For this review, take the finished solid that the model builds, in its own axes (mm). A direction names the side the tool comes from. Give positions to 0.01 mm unless a question says otherwise; leave off trailing zeros. Write each loop counter-clockwise with the first axis right and the second up, starting at its lowest first coordinate (ties: lowest second). Pieces come first, ordered by that corner, then holes. Notation, with made-up numbers: M 76,81.25 L 103,81.25 A28 cw 103,114.25 Z; hole C 24.5,43.25 d3. An arc over 180 degrees is marked long. Use one line per item in the form item = value. Start each with the question number.
Q1. Consider section C-C on x = 49. Write out the cut boundary in (y, z).
Q2. Clearance check with flat-ended pins moving along their axes: pin 1 Ø8 at (x, z) = (40.5, 31) entering from +Y; pin 2 Ø10 at (x, y) = (13.5, 5.5) entering from +Z. State where each tip first meets the part, or that it passes through.
Q3. Consider section A-A on z = 4. Write out the cut boundary in (x, y), and give its area (3 significant figures).
Q4. Consider section D-D on z = 21.5. Write out the cut boundary in (x, y) (1 decimal).
Q5. For probe 1 along Y at (x, z) = (35, 38); probe 2 along Y at (x, z) = (63, 31); probe 3 along X at (y, z) = (28, 43), list the stretches that pass through material, from the lowest coordinate up. Write a range as [from, to].
Q6. Consider section B-B on y = 6. Write out the cut boundary in (x, z).
Q7. Tool access review of faces 1 (the flat face through (55, 40, 34)), 2 (the flat face through (32.36, 24.72, 37.78)), 3 (the flat face through (50, 20, 50)): name each direction out of +Z, -Z, +X, -X, +Y, -Y from which nothing blocks a thin tool from reaching the whole face with its end or side.
```python
from build123d import *

# Parameters (mm, degrees)
SKETCH1_W            = 70
SKETCH1_H            = 50
BOSS_EXTRUDE1_DEPTH  = 50
CUT_EXTRUDE1_DEPTH   = 50
CUT_EXTRUDE2_DEPTH   = 81
CUT_EXTRUDE4_DEPTH   = 30
BOSS_EXTRUDE4_DEPTH  = 73
SKETCH7_W            = 70
SKETCH7_H            = 50
CUT_EXTRUDE5_DEPTH   = 73
SKETCH8_W            = 70
SKETCH8_H            = 50
CUT_EXTRUDE6_DEPTH   = 73
CUT_EXTRUDE7_DEPTH   = 73
CUT_EXTRUDE8_DEPTH   = 73
CUT_EXTRUDE9_DEPTH   = 73
CUT_EXTRUDE10_DEPTH  = 73
CUT_EXTRUDE11_DEPTH  = 73
CUT_EXTRUDE12_DEPTH  = 73
CUT_EXTRUDE13_DEPTH  = 73
CUT_EXTRUDE14_DEPTH  = 73
CUT_EXTRUDE15_DEPTH  = 73
CUT_EXTRUDE16_DEPTH  = 73
CUT_EXTRUDE17_DEPTH  = 73
BOSS_EXTRUDE6_DEPTH  = 40
BOSS_EXTRUDE9_DEPTH  = 20
CUT_EXTRUDE18_DEPTH  = 20
CUT_EXTRUDE19_DEPTH  = 20
CUT_EXTRUDE20_DEPTH  = 20
CUT_EXTRUDE21_DEPTH  = 20
CUT_EXTRUDE22_DEPTH  = 20
SKETCH28_W           = 25
SKETCH28_H           = 30
BOSS_EXTRUDE10_DEPTH = 20
CUT_EXTRUDE23_DEPTH  = 20
BOSS_EXTRUDE12_DEPTH = 10
CUT_EXTRUDE24_DEPTH  = 10
CUT_EXTRUDE25_DEPTH  = 10
CUT_EXTRUDE28_DEPTH  = 10
BOSS_EXTRUDE14_DEPTH = 35


with BuildPart() as part:
    # Sketch1 → Boss-Extrude1 (new body)
    with BuildSketch(Plane.XY):
        with Locations((35, 25)):
            Rectangle(SKETCH1_W, SKETCH1_H)
    extrude(amount=BOSS_EXTRUDE1_DEPTH)

    # Sketch2 → Cut-Extrude1 (cut)
    with BuildSketch(Plane.XY.offset(50)):
        Polygon((20, 50), (0, 30), (0, 50), align=None)
    extrude(amount=-CUT_EXTRUDE1_DEPTH, mode=Mode.SUBTRACT)

    # Sketch3 → Cut-Extrude2 (cut)
    with BuildSketch(Plane(origin=(70, 0, 0), x_dir=(0, 0, -1), z_dir=(1, 0, 0))):
        Polygon((-50, 40), (-20, 40), (-10, 50), (-50, 50), align=None)
    extrude(amount=-CUT_EXTRUDE2_DEPTH, mode=Mode.SUBTRACT)

    # Sketch4 → Cut-Extrude4 (cut)
    with BuildSketch(Plane.XY.offset(50)):
        Polygon((0, 0), (20, 0), (40, 40), (10, 40), (0, 30), align=None)
    extrude(amount=-CUT_EXTRUDE4_DEPTH, mode=Mode.SUBTRACT)

    # Sketch6 → Boss-Extrude4 (add)
    with BuildSketch(Plane(origin=(0, 24.390243902, 30.487804878), x_dir=(1, 0, 0), z_dir=(0, 0.624695048, 0.780868809))):
        Polygon((20, -31.234752378), (70, 32.796489997), (20, 32.796489997), align=None)
        Polygon((20, -31.234752378), (20, 32.796489997), (0, -31.234752378), align=None)
    extrude(amount=-BOSS_EXTRUDE4_DEPTH)

    # Sketch7 → Cut-Extrude5 (cut)
    with BuildSketch(Plane.XZ):
        with Locations((35, 25)):
            Rectangle(SKETCH7_W, SKETCH7_H)
    extrude(amount=CUT_EXTRUDE5_DEPTH, mode=Mode.SUBTRACT)

    # Sketch8 → Cut-Extrude6 (cut)
    with BuildSketch(Plane(origin=(0, 0, 0), x_dir=(-1, 0, 0), z_dir=(0, 0, -1))):
        with Locations((-35, 25)):
            Rectangle(SKETCH8_W, SKETCH8_H)
    extrude(amount=CUT_EXTRUDE6_DEPTH, mode=Mode.SUBTRACT)

    # Sketch9 → Cut-Extrude7 (cut)
    with BuildSketch(Plane.XY):
        Polygon((9.756097561, 0), (0, -40), (20, -40), (44.390243902, 0), align=None)
    extrude(amount=-CUT_EXTRUDE7_DEPTH, mode=Mode.SUBTRACT)

    # Sketch10 → Cut-Extrude8 (cut)
    with BuildSketch(Plane(origin=(32.359063313, -19.731136167, 0), x_dir=(0, 0, 1), z_dir=(-0.853796176, 0.520607424, 0))):
        Polygon((0, 23.109890541), (0, -23.739698546), (-11.485613867, -23.739698546), (-43.485613867, 23.109890541), align=None)
    extrude(amount=-CUT_EXTRUDE8_DEPTH, mode=Mode.SUBTRACT)

    # Sketch11 → Cut-Extrude9 (cut)
    with BuildSketch(Plane(origin=(0, 24.390243902, 30.487804878), x_dir=(1, 0, 0), z_dir=(0, 0.624695048, 0.780868809))):
        Polygon((0, -31.234752378), (20, -31.234752378), (70, 32.796489997), (20, 32.796489997), (0, 4.685212857), align=None)
    extrude(amount=CUT_EXTRUDE9_DEPTH, mode=Mode.SUBTRACT)

    # Sketch12 → Cut-Extrude10 (cut)
    with BuildSketch(Plane(origin=(-2.213114754, 1.229508197, -0.983606557), x_dir=(0.316569925, -0.17587218, -0.932122556), z_dir=(0.814821714, -0.45267873, 0.362142984))):
        Polygon((-22.511639083, 36.962823095), (-11.783436083, 53.42072243), (-22.511639083, 39.822720357), align=None)
    extrude(amount=-CUT_EXTRUDE10_DEPTH, mode=Mode.SUBTRACT)

    # Sketch13 → Cut-Extrude11 (cut)
    with BuildSketch(Plane(origin=(-7.126507887, 3.959171049, 20.983606557), x_dir=(-0.948569177, -0.058694552, -0.311081126), z_dir=(0.316569925, -0.17587218, -0.932122556))):
        Polygon((-18.055096359, 35.598308966), (-15.837888954, 33.59045957), (-16.59090279, 33.141654832), align=None)
    extrude(amount=-CUT_EXTRUDE11_DEPTH, mode=Mode.SUBTRACT)

    # Sketch14 → Cut-Extrude12 (cut)
    with BuildSketch(Plane(origin=(17.950733753, 32.311320755, 0), x_dir=(0.874157276, -0.485642931, 0), z_dir=(0.485642931, 0.874157276, 0))):
        Polygon((-11.501257989, -19.682539683), (-10.684144486, -20), (-11.501257989, -20), align=None)
    extrude(amount=-CUT_EXTRUDE12_DEPTH, mode=Mode.SUBTRACT)

    # Sketch15 → Cut-Extrude13 (cut)
    with BuildSketch(Plane(origin=(0, 0, 0), x_dir=(1, 0, 0), z_dir=(0, 1, 0))):
        Polygon((44.390243902, 43.485613867), (44.390243902, 0), (65.602738471, 43.485613867), align=None)
    extrude(amount=-CUT_EXTRUDE13_DEPTH, mode=Mode.SUBTRACT)

    # Sketch16 → Cut-Extrude14 (cut)
    with BuildSketch(Plane(origin=(0, -40, 0), x_dir=(1, 0, 0), z_dir=(0, 1, 0))):
        Polygon((20, 11.485613867), (20, 0), (0, 0), (2.241095389, 11.485613867), align=None)
    extrude(amount=-CUT_EXTRUDE14_DEPTH, mode=Mode.SUBTRACT)

    # Sketch17 → Cut-Extrude15 (cut)
    with BuildSketch(Plane(origin=(0, 0, 0), x_dir=(0.191510359, 0, -0.981490592), z_dir=(0.981490592, 0, 0.191510359))):
        Polygon((11.702214937, -40), (7.135496913, -45.602738471), (0, -40), align=None)
    extrude(amount=-CUT_EXTRUDE15_DEPTH, mode=Mode.SUBTRACT)

    # Sketch18 → Cut-Extrude16 (cut)
    with BuildSketch(Plane.ZY.offset(-20)):
        Polygon((-7.003423089, -45.602738471), (0, -40), (-11.485613867, -40), align=None)
    extrude(amount=-CUT_EXTRUDE16_DEPTH, mode=Mode.SUBTRACT)

    # Sketch19 → Cut-Extrude17 (cut)
    with BuildSketch(Plane(origin=(0, -24.390243902, 19.512195122), x_dir=(1, 0, 0), z_dir=(0, -0.780868809, 0.624695048))):
        Polygon((0, -33.956559528), (1.366521578, -33.956559528), (0, -24.987801902), align=None)
    extrude(amount=-CUT_EXTRUDE17_DEPTH, mode=Mode.SUBTRACT)

    # Sketch20 → Boss-Extrude6 (add)
    with BuildSketch(Plane.XY.offset(50)):
        Polygon((20, 0), (70, 0), (70, 40), (40, 40), align=None)
    extrude(amount=-BOSS_EXTRUDE6_DEPTH)

    # Sketch22 → Boss-Extrude9 (add)
    with BuildSketch(Plane.ZY):
        Polygon((20, 0), (50, 0), (20, 50), align=None)
    extrude(amount=-BOSS_EXTRUDE9_DEPTH)

    # Sketch23 → Cut-Extrude18 (cut)
    with BuildSketch(Plane(origin=(0, 24.390243902, 30.487804878), x_dir=(1, 0, 0), z_dir=(0, 0.624695048, 0.780868809))):
        Polygon((0, -31.234752378), (20, 32.796489997), (20, -31.234752378), align=None)
    extrude(amount=CUT_EXTRUDE18_DEPTH, mode=Mode.SUBTRACT)

    # Sketch24 → Cut-Extrude19 (cut)
    with BuildSketch(Plane(origin=(0, 24.390243902, 30.487804878), x_dir=(1, 0, 0), z_dir=(0, 0.624695048, 0.780868809))):
        Polygon((20, 32.796489997), (20, -31.234752378), (0, -31.234752378), (0, 0), align=None)
    extrude(amount=CUT_EXTRUDE19_DEPTH, mode=Mode.SUBTRACT)

    # Sketch25 → Cut-Extrude20 (cut)
    with BuildSketch(Plane(origin=(0, 0, 0), x_dir=(0.293651999, -0.139834285, -0.945629354), z_dir=(0.85377141, -0.406557814, 0.325246251))):
        Polygon((-35.72624266, 24.401635644), (-32.240755571, 22.020988264), (-21.149935654, 38.258970398), (-21.149935654, 52.103855338), align=None)
    extrude(amount=-CUT_EXTRUDE20_DEPTH, mode=Mode.SUBTRACT)

    # Sketch26 → Cut-Extrude21 (cut)
    with BuildSketch(Plane(origin=(0, 0, 20), x_dir=(-1, 0, 0), z_dir=(0, 0, -1))):
        Polygon((0, 30), (0, 37.5), (-7.5, 37.5), align=None)
    extrude(amount=-CUT_EXTRUDE21_DEPTH, mode=Mode.SUBTRACT)

    # Sketch27 → Cut-Extrude22 (cut)
    with BuildSketch(Plane(origin=(-2.564728872, 23.387884709, 35.967269174), x_dir=(-0.998217939, -0.032530406, -0.050027178), z_dir=(0.059673661, -0.54416696, -0.836852062))):
        Polygon((-2.569307534, 16.733584836), (-2.569307534, 29.52608638), (-18.788687646, 31.014533667), (-9.963436703, 16.446669873), align=None)
    extrude(amount=-CUT_EXTRUDE22_DEPTH, mode=Mode.SUBTRACT)

    # Sketch28 → Boss-Extrude10 (add)
    with BuildSketch(Plane.ZY):
        with Locations((12.5, 15)):
            Rectangle(SKETCH28_W, SKETCH28_H)
    extrude(amount=-BOSS_EXTRUDE10_DEPTH)

    # Sketch29 → Cut-Extrude23 (cut)
    with BuildSketch(Plane(origin=(0, 0, 20), x_dir=(-1, 0, 0), z_dir=(0, 0, -1))):
        Polygon((0, 48.224543081), (0, 50), (-16.19047619, 50), align=None)
    extrude(amount=-CUT_EXTRUDE23_DEPTH, mode=Mode.SUBTRACT)

    # Sketch30 → Boss-Extrude12 (add)
    with BuildSketch(Plane(origin=(0, 24.390243902, 30.487804878), x_dir=(1, 0, 0), z_dir=(0, 0.624695048, 0.780868809))):
        Polygon((20, 32.796489997), (0, 7.183993047), (19.391822061, 9.570105394), align=None)
    extrude(amount=-BOSS_EXTRUDE12_DEPTH)

    # Sketch31 → Cut-Extrude24 (cut)
    with BuildSketch(Plane(origin=(-2.564728872, 23.387884709, 35.967269174), x_dir=(-0.998217939, -0.032530406, -0.050027178), z_dir=(0.059673661, -0.54416696, -0.836852062))):
        Polygon((-9.678751188, 15.976738782), (-2.569307534, 7.787398424), (-2.569307534, 4.241162369), align=None)
    extrude(amount=-CUT_EXTRUDE24_DEPTH, mode=Mode.SUBTRACT)

    # Sketch32 → Cut-Extrude25 (cut)
    with BuildSketch(Plane(origin=(0, 37.5, 0), x_dir=(-1, 0, 0), z_dir=(0, -1, 0))):
        Polygon((-7.380952381, -27.5), (0, -26.973684211), (0, -27.5), align=None)
    extrude(amount=-CUT_EXTRUDE25_DEPTH, mode=Mode.SUBTRACT)

    # Sketch35 → Cut-Extrude28 (cut)
    with BuildSketch(Plane(origin=(0, 24.390243902, 30.487804878), x_dir=(1, 0, 0), z_dir=(0, 0.624695048, 0.780868809))):
        Polygon((70, 32.796489997), (70, -31.234752378), (0, -31.234752378), align=None)
    extrude(amount=CUT_EXTRUDE28_DEPTH, mode=Mode.SUBTRACT)

    # Sketch36 → Boss-Extrude14 (add)
    with BuildSketch(Plane.XY.offset(50)):
        Polygon((70, 0), (70, 16.007810594), (28.003905297, 16.007810594), (20, 0), align=None)
        Polygon((40, 40), (28.003905297, 16.007810594), (70, 16.007810594), (70, 40), align=None)
    extrude(amount=-BOSS_EXTRUDE14_DEPTH)


solid = part.part
```
Working result:
q1.outline = M 0,0 L 50,0 L 50,10 L 40,18 L 40,50 L 0,50 Z
q2.pin_1 = 40
q2.pin_2 = 49.6
q3.outline = M 0,0 L 70,0 L 70,50 L 20,50 L 0,30 Z
q3.area = 3,300 mm²
q4.outline = M 0,0 L 70,0 L 70,40 L 40,40 L 37.8,35.6 L 5.6,35.6 L 0,30 Z
q5.probe_1 = [0, 30]
q5.probe_2 = [0, 40]
q5.probe_3 = [34, 70]
q6.outline = M 0,0 L 70,0 L 70,50 L 23,50 L 23,45.2 L 0,45.2 Z
q7.face_1 = +Z, +X, -X, +Y
q7.face_2 = +Z, -X, +Y
q7.face_3 = +Z, +X, -X, +Y, -Y
